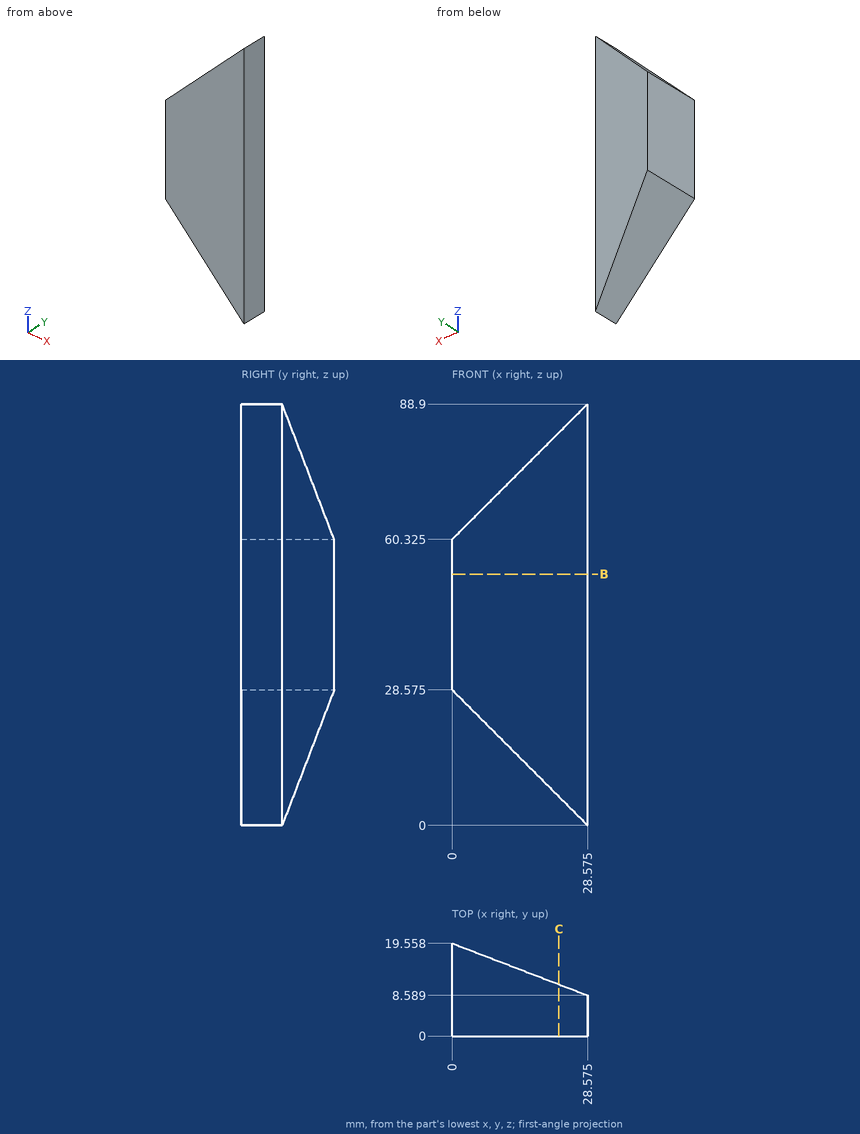
Here's the drawing with two shaded views (mm, measured from the low corner). I have some questions. Coordinates: 2 decimals unless noted, no trailing zeros. Write each loop counter-clockwise with the first axis right and the second up, starting at its lowest first coordinate (ties: lowest second). Pieces come first, ordered by that corner, then holes.
Item 1: If I drill on line 1 (Y direction, x = 27.5, z = 34); line 2 (Y direction, x = 4.25, z = 63); line 3 (Z direction, x = 21.75, y = 3.5) (1 decimal), over which ranges is the centre line in solid material (lowest first)?
Item 2: I want a section at B-B on z = 53. Write out the boundary of the cut face in (x, y) (3 decimals).
Item 3: I want a section at C-C on x = 22.5. Write out the boundary of the cut face in (y, z) (3 decimals).
Item 4: Will these pins go through, and if not, where does the flat tip stop? pin 1 (1.5 mm diameter, centred on x = 13, z = 70, fed in from +Y); pin 2 (5 mm diameter, centred on y = 14.5, z = 73, fed in from -X) (1 decimal); pin 3 (6 mm diameter, centred on x = 22.5, z = 47.5, fed in from +Y).
Findings below:
1. line 1: y = 0 to 9
1. line 2: y = 0 to 17.93
1. line 3: z = 6.8 to 82.1
2. outline: (0, 0) - (28.575, 0) - (28.575, 8.589) - (0, 19.558) - close
3. outline: (0, 6.075) - (10.921, 6.075) - (10.921, 82.825) - (0, 82.825) - close
4. pin 1: stops at y = 14.86
4. pin 2: stops at x = 10.2
4. pin 3: stops at y = 12.07
